from build123d import *

# Parameters (mm, degrees)
F0_W      = 96.012
F0_H      = 56.896
F1_DEPTH  = 50.8
F3_DEPTH  = 96.012
F5_DEPTH  = 31.75
F7_DEPTH  = 25.4
F8_W      = 28.956
F8_H      = 11.43
F9_DEPTH  = 59.436
F11_DEPTH = 37.084
F12_R     = 7.9375
F13_DEPTH = 25.4


with BuildPart() as f1:
    # F0 (on Top) → F1 (new body)
    with BuildSketch(Plane.XY):
        Rectangle(F0_W, F0_H)
    extrude(amount=F1_DEPTH)

    # F2 (on face) → F3 (cut)
    with BuildSketch(Plane.YZ.offset(48.006)):
        Polygon((-28.448, 6.604), (15.748, 50.8), (-28.448, 50.8), align=None)
    extrude(amount=-F3_DEPTH, mode=Mode.SUBTRACT)

    # F4 (on face) → F5 (cut)
    with BuildSketch(Plane(origin=(0, 28.448, 0), x_dir=(-1, 0, 0), z_dir=(0, 1, 0))):
        Polygon((-48.006, 32.004), (-29.21, 50.8), (-48.006, 50.8), align=None)
    extrude(amount=-F5_DEPTH, mode=Mode.SUBTRACT)

    # F6 (on face) → F7 (cut)
    with BuildSketch(Plane.YZ.offset(48.006)):
        Polygon((-9.144, 25.908), (-28.448, 6.604), (-28.448, 0), (-9.144, 0), align=None)
    extrude(amount=-F7_DEPTH, mode=Mode.SUBTRACT)

    # F8 (on face) → F9 (cut)
    with BuildSketch(Plane(origin=(0, 0, 0), x_dir=(1, 0, 0), z_dir=(0, 0, -1))):
        with Locations((-8.128, 22.733)):
            Rectangle(F8_W, F8_H)
    extrude(amount=-F9_DEPTH, mode=Mode.SUBTRACT)

    # F10 (on face) → F11 (cut)
    with BuildSketch(Plane(origin=(0, 28.448, 0), x_dir=(-1, 0, 0), z_dir=(0, 1, 0))):
        Polygon((48.006, 50.8), (-0.762, 50.8), (31.793627, 32.004), (48.006, 32.004), align=None)
    extrude(amount=-F11_DEPTH, mode=Mode.SUBTRACT)

    # F12 (on face) → F13 (cut)
    with BuildSketch(Plane.YZ.offset(48.006)):
        with Locations((9.145532, 14.183054)):
            Circle(F12_R)
    extrude(amount=-F13_DEPTH, mode=Mode.SUBTRACT)


solid = f1.part
Part model, mm, in its own coordinate system. A direction names the side the tool comes from. Give positions to 0.01 mm unless a question says otherwise; leave off trailing zeros. Order: outer loops, then holes, each group sorted by start corner. A loop starts at its lowest first (then second) coordinate and runs counter-clockwise, first axis right, second up. Notation, with made-up numbers: (14.25, 13) - (56.25, 13) arc R32 ccw to (56.25, 48) - close; hole circle Ø8 at (19.5, 8.25). An arc over 180 degrees is marked (long way). One line per question, with ' | ' between items.
1. Band-saw the part on A-A on y = -22.5. List the corners of the cut face in (x, z).
Filled in:
outline: (-48.01, 0) - (-22.61, 0) - (-22.61, 12.55) - (-48.01, 12.55) - close; (6.35, 0) - (22.61, 0) - (22.61, 12.55) - (6.35, 12.55) - close
2. Band-saw the part on B-B on y = 24. List the corners of the cut face in (x, z), then the cut area to 3 significant figures.
Filled in:
outline: (-48.01, 0) - (48.01, 0) - (48.01, 32) - (29.21, 50.8) - (0.76, 50.8) - (-31.79, 32) - (-48.01, 32) - close | area: 4,090 mm²
3. Which spindle directions (+Z, -Z, +X, -X, +Y, -Y) get a long thin tool onto all of the face, cutting with end or side? Do faces 1 (the face through (35.484, 16.716, 16.567)), 2 (the face through (35, -9.144, 13)), 3 (the face through (-1, 28.448, 19)), 4 (the face through (-22.606, -21, 7)). Say none if no direction does.
Filled in:
face 1: +X | face 2: +Z, -Z, +X, -Y | face 3: +Z, -Z, +X, -X, +Y | face 4: +Z, -Z, -Y
4. Pull direction X, two halves, no side cores. Call faces 5 (the face through (-18.905, 16.42, 39.445)), 6 (the face through (22.606, -17, 10)), 7 (the face through (-8, -17.018, 9)), 8 (the face through (-40, 13, 32.004)): +X half, -X half, draft (parallel to the pull), parting line (faces both ways), or undercut.
Filled in:
face 5: -X half | face 6: +X half | face 7: undercut | face 8: draft
5. Band-saw the part on D-D on x = 27. List the corners of the cut face in (y, z) (1 decimal).
Filled in:
outline: (-9.1, 0) - (28.4, 0) - (28.4, 50.8) - (15.7, 50.8) - (-9.1, 25.9) - close; hole circle Ø15.9 at (9.1, 14.2)
6. Drop flat-ended pins along their axis: P1, Ø5, axis at x = -43.5, y = 5.5, coming from the +Z side; P2, Ø9.5, axis at y = -17, z = 14, coming from the +X side; P3, Ø1.5, axis at y = 16, z = 37, coming from the -X side. Give the stop position or say it passes through.
Filled in:
P1: z = 32 | P2: x = 22.61 | P3: x = -24.44
7. Band-saw the part on C-C on x = 4.5. List the corners of the cut face in (y, z).
Filled in:
outline: (-17.02, 0) - (28.45, 0) - (28.45, 50.8) - (15.75, 50.8) - (-17.02, 18.03) - close
8. Drill centre lines: probe 1 along X at (y, z) = (-18, 11); probe 2 along Y at (x, z) = (37, 13.5); probe 3 along Z at (x, y) = (24, 13.5). Where is each one in solid material? Low to high.
Filled in:
probe 1: -48.01 to -22.61, 6.35 to 22.61 | probe 2: -9.14 to 1.24, 17.05 to 28.45 | probe 3: 0 to 7.55, 20.82 to 48.55
